Geometry: final body of the model. Coordinates: model frame, mm. A direction names the side the tool comes from. Coordinates: 2 decimals unless noted, no trailing zeros. Write each loop counter-clockwise with the first axis right and the second up, starting at its lowest first coordinate (ties: lowest second). Pieces come first, ordered by that corner, then holes. Notation, with made-up numbers: (81.5, 20.5) -> (135.5, 20.5) arc R21 cw to (135.5, 24.5) -> close; hole circle Ø4 at (5, 87). An arc over 180 degrees is marked (long way). One line per item, written item: value.
```python
from build123d import *

# Parameters (mm, degrees)
EXTRUDE_1_DEPTH      = 39
SKETCH_2_OUTSIDE_W   = 212.666
SKETCH_2_OUTSIDE_H   = 65.166
SKETCH_2_OUTSIDE_R   = 4.25
CUT_EXTRUDE_2_DEPTH  = 40
CUT_EXTRUDE_4_DEPTH  = 28
CUT_EXTRUDE_7_DEPTH  = 28
CUT_EXTRUDE_9_DEPTH  = 23
CUT_EXTRUDE_10_DEPTH = 28
SKETCH_17_R          = 1.75
CUT_EXTRUDE_13_DEPTH = 2
CUT_EXTRUDE_16_REACH = 41
SKETCH_21_R          = 4.25


with BuildPart() as part:
    # 草图1 → 凸台-拉伸1 (new body)
    with BuildSketch(Plane.XY):
        with BuildLine():
            Line((0, 13.5), (147.5, 13.5))
            ThreePointArc((147.5, 13.5), (161, 0), (147.5, -13.5))
            Line((147.5, -13.5), (0, -13.5))
            ThreePointArc((0, -13.5), (-13.5, 0), (0, 13.5))
        make_face()
    extrude(amount=EXTRUDE_1_DEPTH)

    # 草图2 outside → 切除-拉伸2 (cut, through all)
    with BuildSketch(Plane.XY.offset(39)):
        with Locations((73.75, 0)):
            Rectangle(SKETCH_2_OUTSIDE_W, SKETCH_2_OUTSIDE_H)
        with BuildLine():
            Line((0, -13.5), (147.5, -13.5))
            ThreePointArc((147.5, -13.5), (161, 0), (147.5, 13.5))
            Line((147.5, 13.5), (0, 13.5))
            ThreePointArc((0, 13.5), (-13.5, 0), (0, -13.5))
        make_face(mode=Mode.SUBTRACT)
        with Locations((147.5, 0)):
            Circle(SKETCH_2_OUTSIDE_R)
    extrude(amount=-CUT_EXTRUDE_2_DEPTH, mode=Mode.SUBTRACT)

    # 草图5 → 切除-拉伸4 (cut, through all)
    with BuildSketch(Plane(origin=(0, 13.5, 0), x_dir=(1, 0, 0), z_dir=(0, 1, 0))):
        with BuildLine():
            Line((-32, -37), (17, -37))
            ThreePointArc((17, -37), (27.606601718, -32.606601718), (32, -22))
            Line((32, -22), (32, -17))
            ThreePointArc((32, -17), (27.606601718, -6.393398282), (17, -2))
            Line((17, -2), (-32, -2))
            Line((-32, -2), (-32, -37))
        make_face()
    extrude(amount=-CUT_EXTRUDE_4_DEPTH, mode=Mode.SUBTRACT)

    # 草图11 → 切除-拉伸7 (cut, through all)
    with BuildSketch(Plane.XZ.offset(13.5)):
        with BuildLine():
            Line((108.5, 37), (201.5, 37))
            Line((201.5, 37), (201.5, 2))
            Line((201.5, 2), (108.5, 2))
            ThreePointArc((108.5, 2), (97.893398282, 6.393398282), (93.5, 17))
            Line((93.5, 17), (93.5, 22))
            ThreePointArc((93.5, 22), (97.893398282, 32.606601718), (108.5, 37))
        make_face()
    extrude(amount=-CUT_EXTRUDE_7_DEPTH, mode=Mode.SUBTRACT)

    # 草图14 → 切除-拉伸9 (cut)
    with BuildSketch(Plane(origin=(0, 13.5, 0), x_dir=(1, 0, 0), z_dir=(0, 1, 0))):
        with BuildLine():
            Line((58.944791853, -2.5), (70.944791853, -2.5))
            ThreePointArc((70.944791853, -2.5), (87.944791853, -19.5), (70.944791853, -36.5))
            Line((70.944791853, -36.5), (58.944791853, -36.5))
            ThreePointArc((58.944791853, -36.5), (41.944791853, -19.5), (58.944791853, -2.5))
        make_face()
    extrude(amount=-CUT_EXTRUDE_9_DEPTH, mode=Mode.SUBTRACT)

    # 草图16 → 切除-拉伸10 (cut, through all)
    with BuildSketch(Plane.XZ.offset(13.5)):
        with BuildLine():
            Line((62, 29), (70, 29))
            ThreePointArc((70, 29), (79.5, 19.5), (70, 10))
            Line((70, 10), (62, 10))
            ThreePointArc((62, 10), (52.5, 19.5), (62, 29))
        make_face()
    extrude(amount=-CUT_EXTRUDE_10_DEPTH, mode=Mode.SUBTRACT)

    # 草图17 → 切除-拉伸13 (cut)
    with BuildSketch(Plane(origin=(0, 0, 0), x_dir=(-1, 0, 0), z_dir=(0, 0, -1))):
        with Locations((-4.949747468, 4.949747468)):
            Circle(SKETCH_17_R)
        with Locations((4.949747468, 4.949747468)):
            Circle(SKETCH_17_R)
        with Locations((-4.949747468, -4.949747468)):
            Circle(SKETCH_17_R)
        with Locations((4.949747468, -4.949747468)):
            Circle(SKETCH_17_R)
        Circle(SKETCH_17_R)
    extrude(amount=-CUT_EXTRUDE_13_DEPTH, mode=Mode.SUBTRACT)

    # 草图21 → 切除-拉伸16 (cut, up to next)
    with BuildSketch(Plane.XY.offset(39), mode=Mode.PRIVATE) as cut_extrude_16_sk1:
        Circle(SKETCH_21_R)
    cut_extrude_16_tool1 = extrude(cut_extrude_16_sk1.sketch, amount=-CUT_EXTRUDE_16_REACH, mode=Mode.PRIVATE) & part.part
    add(cut_extrude_16_tool1.solids().sort_by_distance((0, 0, 39))[0], mode=Mode.SUBTRACT)


solid = part.part
```
(1) Reachability of faces 4 (the flat face through (134, 0, 37)), 5 (the cylindrical face through (2.285, 3.584, 38.014)), 6 (the flat face through (65, 2, 2.5)), 7 (the cylindrical face through (52.502, -11.528, 19.291)), 8 (the cylindrical face through (27.49, 0.19, 32.72)) from +Z, -Z, +X, -X, +Y, -Y: full face, straight path, thin tool, end or side. Return the list, or none.
Responses:
face 4: +X, +Y, -Y
face 5: +Z
face 6: +Y
face 7: +Y, -Y
face 8: -X, +Y, -Y
(2) First-contact query: pin 1 (5 mm diameter, centred on y = 1, z = 20, fed in from -X); pin 2 (3 mm diameter, centred on y = 7, z = 10.5, fed in from -X); pin 3 (2 mm diameter, centred on y = 1.5, z = 5, fed in from -X). Flat tips, straight axial feed; report the tip coordinate or a pass-through.
Responses:
pin 1: stops at x = 31.99
pin 2: stops at x = 29.69
pin 3: stops at x = 24.48
(3) Pull-direction query (Z, two-part tool) for faces 1 (the flat face through (75, 0, 39)), 2 (the flat face through (5, 0, 37)), 3 (the cylindrical face through (-4.57, 3.24, 0.99)); classes: released by +Z, released by -Z, zero draft, split by the parting line, or undercut.
Responses:
face 1: released by +Z
face 2: undercut
face 3: zero draft
(4) Section B-B (x = 96). Return the cut outline in (y, z).
Responses:
outline: (-13.5, 0) -> (13.5, 0) -> (13.5, 8.71) -> (-13.5, 8.71) -> close; (-13.5, 30.29) -> (13.5, 30.29) -> (13.5, 39) -> (-13.5, 39) -> close
(5) Section C-C (y = 0). State how many separate pieces and enclosed holes the cut face has, then the cut area to 3 significant figures.
Responses:
separate pieces: 5
enclosed holes: 1
area: 1,670 mm2
(6) Section A-A (z = 19.5). Return the cut outline in (x, y), then the cut area to 4 significant figures.
Responses:
outline: (32, -13.5) -> (52.5, -13.5) -> (52.5, -9.5) -> (41.94, -9.5) -> (41.94, 13.5) -> (32, 13.5) -> close; (79.5, -13.5) -> (93.5, -13.5) -> (93.5, 13.5) -> (87.94, 13.5) -> (87.94, -9.5) -> (79.5, -9.5) -> close
area: 494.5 mm2
(7) Section D-D (z = 4.5). Return the cut outline in (x, y), then the cut area to 3 significant figures.
Responses:
outline: (25.29, -13.5) -> (100.21, -13.5) -> (100.21, 13.5) -> (78.94, 13.5) -> (78.94, -9.5) -> (50.94, -9.5) -> (50.94, 13.5) -> (25.29, 13.5) -> close
area: 1,380 mm2
(8) Line query: line 1 (Z direction, x = 64.5, y = 3); line 2 (X direction, y = -10.5, z = 20); line 3 (Z direction, x = 131, y = -9.75). Output: solid intervals per line, ascending. Write a range as [from, to].
Responses:
line 1: z = [0, 2.5], [36.5, 39]
line 2: x = [32, 52.51], [79.49, 93.5]
line 3: z = [0, 2], [37, 39]
